Read the model definition and answer for the solid it produces. Units are mm, in the model's axes. Face numbers are marked on the shaded views. Coordinates: 2 decimals unless noted, no trailing zeros. Order: outer loops, then holes, each group sorted by start corner. A loop starts at its lowest first (then second) coordinate and runs counter-clockwise, first axis right, second up. Notation, with made-up numbers: (86, 20.25) -> (138, 20.25) arc R10 cw to (138, 28.25) -> close; hole circle Ø2 at (84, 32). An arc over 180 degrees is marked (long way). Answer as a JSON object with one key per item and string values. Group by question number.
1) Consider L1, parallel to Y at x = 30, z = -18.8; L2, parallel to Y at x = 106, z = -17.65; L3, parallel to Z at x = 106.5, y = 27.5. Determine where each line is inside the solid, lowest interval first.
2) Section B-B on x = 44 is taken. Determine the outline of the cut face in (y, z), and give its area (3 significant figures).
3) Section D-D on y = -22.05 is taken. Determine the outline of the cut face in (x, z) (3 decimals).
4) Determine the mould class of the marked faces 1 and 2 for opening direction X: released by +X, released by -X, zero draft, split by the parting line, or undercut.
5) Section A-A on y = 37.5 is taken. Determine the outline of the cut face in (x, z).
6) Section C-C on x = 106 is taken. Determine the outline of the cut face in (y, z).
7) Given pin 1 (1.5 mm diameter, centred on y = -34, z = -18.5, fed in from +X); pin 2 (9 mm diameter, centred on x = 44, y = -30, fed in from +Z); pin 3 (5 mm diameter, centred on x = 51, z = -6, fed in from -Y), each flat-ended and moving along its own axis, determine where each tip first touches the part or whether it passes through.
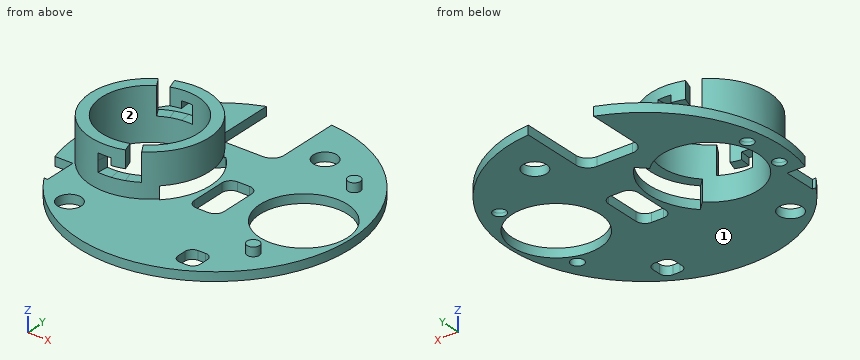
from build123d import *

# Parameters (mm, degrees)
SKETCH1_R                                           = 46
CAGE_PLATE_DEPTH                                    = 3
SKETCH2_R                                           = 20
SKETCH2_R_2                                         = 16.25
BAYONET_SOCKET_DEPTH                                = 14.5
SKETCH3_R                                           = 2.075
TURBIDITY_EAR_PINS_DEPTH                            = 3
HUB_BORE_AND_TURBIDITY_BORE_DEPTH                   = 127.008928255
HUB_BORE_AND_TURBIDITY_BORE_DEPTH_BACK              = 127.008928255
SKETCH4_R                                           = 16.25
SKETCH4_R_2                                         = 14.8
TDS_NOTCH_DS_HOLE_FLOW_WINDOW_HOSE_NOTCH_DEPTH      = 127.008928255
TDS_NOTCH_DS_HOLE_FLOW_WINDOW_HOSE_NOTCH_DEPTH_BACK = 127.008928255
SKETCH5_R                                           = 4
SKETCH5_W                                           = 12
SKETCH5_H                                           = 11
SKETCH6_R                                           = 2.15
POST_PIN_SOCKETS_BLIND_DEPTH                        = 1.6
HUB_CABLE_WINDOW_DEPTH                              = 3.75
J_ENTRY_SLOTS_DEPTH                                 = 4.95
J_TWIST_CHANNELS_DEPTH                              = 1.8
J_LOCK_NOTCHES_DEPTH                                = 3


with BuildPart() as part:
    # Sketch1 → Cage_plate (new body)
    with BuildSketch(Plane.XY.offset(-19.5)):
        with Locations((70, 0)):
            Circle(SKETCH1_R)
    extrude(amount=CAGE_PLATE_DEPTH)

    # Sketch2 → Bayonet_socket (add)
    with BuildSketch(Plane.XY.offset(-16.5)):
        with Locations(Location((48, 0, 0), (0, 0, 180))):
            Circle(SKETCH2_R)
        with Locations(Location((48, 0, 0), (0, 0, 180))):
            Circle(SKETCH2_R_2, mode=Mode.SUBTRACT)
    extrude(amount=BAYONET_SOCKET_DEPTH)

    # Sketch3 → Turbidity_ear_pins (add)
    with BuildSketch(Plane.XY.offset(-16.5)):
        with Locations((100, 22.05)):
            Circle(SKETCH3_R)
        with Locations((100, -22.05)):
            Circle(SKETCH3_R)
    extrude(amount=TURBIDITY_EAR_PINS_DEPTH)

    # Sketch4 → Hub_bore_and_turbidity_bore (cut, two sides: drawn at the far end of the back side and taken through both)
    with BuildSketch(Plane.XY.offset(-19.5).offset(-HUB_BORE_AND_TURBIDITY_BORE_DEPTH_BACK)):
        with Locations((48, 0)):
            Circle(SKETCH4_R)
        with Locations((100, 0)):
            Circle(SKETCH4_R_2)
    extrude(amount=HUB_BORE_AND_TURBIDITY_BORE_DEPTH + HUB_BORE_AND_TURBIDITY_BORE_DEPTH_BACK, mode=Mode.SUBTRACT)

    # Sketch5 → TDS_notch_DS_hole_flow_window_hose_notch (cut, two sides: drawn at the far end of the back side and taken through both)
    with BuildSketch(Plane.XY.offset(-19.5).offset(-TDS_NOTCH_DS_HOLE_FLOW_WINDOW_HOSE_NOTCH_DEPTH_BACK)):
        with Locations((84, 30)):
            Circle(SKETCH5_R)
        with Locations((44, -30)):
            Circle(SKETCH5_R)
        with BuildLine():
            Line((58, 21), (70, 21))
            ThreePointArc((70, 21), (72.828427125, 22.171572875), (74, 25))
            Line((74, 25), (74, 46))
            ThreePointArc((74, 46), (72.828427125, 48.828427125), (70, 50))
            Line((70, 50), (58, 50))
            ThreePointArc((58, 50), (55.171572875, 48.828427125), (54, 46))
            Line((54, 46), (54, 25))
            ThreePointArc((54, 25), (55.171572875, 22.171572875), (58, 21))
        make_face()
        with BuildLine():
            Line((87.5, -38), (90, -38))
            ThreePointArc((90, -38), (91.767766953, -37.267766953), (92.5, -35.5))
            Line((92.5, -35.5), (92.5, -32.5))
            ThreePointArc((92.5, -32.5), (91.767766953, -30.732233047), (90, -30))
            Line((90, -30), (87.5, -30))
            ThreePointArc((87.5, -30), (85.732233047, -30.732233047), (85, -32.5))
            Line((85, -32.5), (85, -35.5))
            ThreePointArc((85, -35.5), (85.732233047, -37.267766953), (87.5, -38))
        make_face()
        with BuildLine():
            Line((73, -12), (77, -12))
            ThreePointArc((77, -12), (79.121320344, -11.121320344), (80, -9))
            Line((80, -9), (80, 3))
            ThreePointArc((80, 3), (79.121320344, 5.121320344), (77, 6))
            Line((77, 6), (73, 6))
            ThreePointArc((73, 6), (70.878679656, 5.121320344), (70, 3))
            Line((70, 3), (70, -9))
            ThreePointArc((70, -9), (70.878679656, -11.121320344), (73, -12))
        make_face()
        with Locations((26, -18.5)):
            Rectangle(SKETCH5_W, SKETCH5_H)
    extrude(amount=TDS_NOTCH_DS_HOLE_FLOW_WINDOW_HOSE_NOTCH_DEPTH + TDS_NOTCH_DS_HOLE_FLOW_WINDOW_HOSE_NOTCH_DEPTH_BACK, mode=Mode.SUBTRACT)

    # Sketch6 → Post_pin_sockets_blind (cut, symmetric)
    with BuildSketch(Plane.XY.offset(-18.4)):
        with Locations((30, 7)):
            Circle(SKETCH6_R)
        with Locations((30, -7)):
            Circle(SKETCH6_R)
        with Locations((106, 17)):
            Circle(SKETCH6_R)
        with Locations((106, -17)):
            Circle(SKETCH6_R)
    extrude(amount=POST_PIN_SOCKETS_BLIND_DEPTH, both=True, mode=Mode.SUBTRACT)

    # Sketch7 → Hub_cable_window (cut, symmetric)
    with BuildSketch(Plane.XY.offset(-16.25)):
        with BuildLine():
            Line((59.207642482, -11.207642482), (62.495689014, -14.495689014))
            ThreePointArc((62.495689014, -14.495689014), (68.5, 0), (62.495689014, 14.495689014))
            Line((62.495689014, 14.495689014), (59.207642482, 11.207642482))
            ThreePointArc((59.207642482, 11.207642482), (63.85, 0), (59.207642482, -11.207642482))
        make_face()
    extrude(amount=HUB_CABLE_WINDOW_DEPTH, both=True, mode=Mode.SUBTRACT)

    # Sketch8 → J_entry_slots (cut, symmetric)
    with BuildSketch(Plane.XY.offset(-6.45)):
        with BuildLine():
            Line((42.928546982, 15.069517719), (41.461334159, 19.429252405))
            ThreePointArc((41.461334159, 19.429252405), (39.336325634, 18.579309634), (37.319302547, 17.497791344))
            Line((37.319302547, 17.497791344), (39.715946854, 13.571457677))
            ThreePointArc((39.715946854, 13.571457677), (41.280369638, 14.410293814), (42.928546982, 15.069517719))
        make_face()
        with BuildLine():
            Line((53.071453018, -15.069517719), (54.538665841, -19.429252405))
            ThreePointArc((54.538665841, -19.429252405), (56.663674366, -18.579309634), (58.680697453, -17.497791344))
            Line((58.680697453, -17.497791344), (56.284053146, -13.571457677))
            ThreePointArc((56.284053146, -13.571457677), (54.719630362, -14.410293814), (53.071453018, -15.069517719))
        make_face()
    extrude(amount=J_ENTRY_SLOTS_DEPTH, both=True, mode=Mode.SUBTRACT)

    # Sketch9 → J_twist_channels (cut, symmetric)
    with BuildSketch(Plane.XY.offset(-9.6)):
        with BuildLine():
            Line((49.772356022, 15.800909915), (50.28511311, 20.372242343))
            ThreePointArc((50.28511311, 20.372242343), (43.562987914, 20.014068146), (37.319302547, 17.497791344))
            Line((37.319302547, 17.497791344), (39.715946854, 13.571457677))
            ThreePointArc((39.715946854, 13.571457677), (44.558610138, 15.523106513), (49.772356022, 15.800909915))
        make_face()
        with BuildLine():
            Line((46.227643978, -15.800909915), (45.71488689, -20.372242343))
            ThreePointArc((45.71488689, -20.372242343), (52.437012086, -20.014068146), (58.680697453, -17.497791344))
            Line((58.680697453, -17.497791344), (56.284053146, -13.571457677))
            ThreePointArc((56.284053146, -13.571457677), (51.441389862, -15.523106513), (46.227643978, -15.800909915))
        make_face()
    extrude(amount=J_TWIST_CHANNELS_DEPTH, both=True, mode=Mode.SUBTRACT)

    # Sketch10 → J_lock_notches (cut, symmetric)
    with BuildSketch(Plane.XY.offset(-8.4)):
        with BuildLine():
            Line((49.772356022, 15.800909915), (50.28511311, 20.372242343))
            ThreePointArc((50.28511311, 20.372242343), (48, 20.5), (45.71488689, 20.372242343))
            Line((45.71488689, 20.372242343), (46.227643978, 15.800909915))
            ThreePointArc((46.227643978, 15.800909915), (48, 15.9), (49.772356022, 15.800909915))
        make_face()
        with BuildLine():
            Line((46.227643978, -15.800909915), (45.71488689, -20.372242343))
            ThreePointArc((45.71488689, -20.372242343), (48, -20.5), (50.28511311, -20.372242343))
            Line((50.28511311, -20.372242343), (49.772356022, -15.800909915))
            ThreePointArc((49.772356022, -15.800909915), (48, -15.9), (46.227643978, -15.800909915))
        make_face()
    extrude(amount=J_LOCK_NOTCHES_DEPTH, both=True, mode=Mode.SUBTRACT)


solid = part.part
Worked answers:
{
 "1": {"L1": "y = -13 to -9.15, -4.85 to 4.85, 9.15 to 22.72", "L2": "y = -28.64 to -19.15, -14.85 to -13.53, 13.53 to 14.85, 19.15 to 28.64", "L3": "z = -19.5 to -16.5"},
 "2": {"outline": "(-37.95, -19.5) -> (-34, -19.5) -> (-34, -16.5) -> (-37.95, -16.5) -> close; (-26, -19.5) -> (-15.75, -19.5) -> (-15.75, -2) -> (-19.6, -2) -> (-19.6, -16.5) -> (-26, -16.5) -> close; (15.75, -19.5) -> (37.95, -19.5) -> (37.95, -16.5) -> (19.6, -16.5) -> (19.6, -11.4) -> (15.75, -11.4) -> close; (15.75, -7.8) -> (19.6, -7.8) -> (19.6, -2) -> (15.75, -2) -> close", "area": "207 mm²"},
 "3": {"outline": "(32, -19.5) -> (110.371, -19.5) -> (110.371, -16.5) -> (102.075, -16.5) -> (102.075, -13.5) -> (97.925, -13.5) -> (97.925, -16.5) -> (32, -16.5) -> close"},
 "4": {"face 1": "zero draft", "face 2": "undercut"},
 "5": {"outline": "(43.36, -19.5) -> (54, -19.5) -> (54, -16.5) -> (43.36, -16.5) -> close; (74, -19.5) -> (96.64, -19.5) -> (96.64, -16.5) -> (74, -16.5) -> close"},
 "6": {"outline": "(-28.64, -19.5) -> (-19.15, -19.5) -> (-19.15, -16.8) -> (-14.85, -16.8) -> (-14.85, -19.5) -> (-13.53, -19.5) -> (-13.53, -16.5) -> (-28.64, -16.5) -> close; (13.53, -19.5) -> (14.85, -19.5) -> (14.85, -16.8) -> (19.15, -16.8) -> (19.15, -19.5) -> (28.64, -19.5) -> (28.64, -16.5) -> (13.53, -16.5) -> close"},
 "7": {"pin 1": "stops at x = 101.79", "pin 2": "stops at z = -16.5", "pin 3": "stops at y = -19.99"}
}
